```python
from build123d import *

# Parameters (mm, degrees)
SKETCH_1_R          = 8.9
SKETCH_1_R_2        = 1.5
EXTRUDE_1_DEPTH     = 3.5
SKETCH_2_R          = 7.6
CUT_EXTRUDE_1_DEPTH = 0.5
SKETCH_3_R          = 2
EXTRUDE_2_DEPTH     = 13
SKETCH_8_R          = 4
EXTRUDE_4_DEPTH     = 10
CUT_EXTRUDE_START   = -11.5
SKETCH_13_R         = 4
CUT_EXTRUDE_3_DEPTH = 11.5
SKETCH_16_R         = 8.9
SKETCH_16_R_2       = 2
CUT_EXTRUDE_5_DEPTH = 1
SKETCH_17_R         = 2
EXTRUDE_5_DEPTH     = 2


with BuildPart() as part:
    # 草图1 → 凸台-拉伸1 (new body)
    with BuildSketch(Plane.XY):
        Circle(SKETCH_1_R)
        with Locations((0, 5.075)):
            Circle(SKETCH_1_R_2, mode=Mode.SUBTRACT)
        with Locations((4.395078924, -2.5375)):
            Circle(SKETCH_1_R_2, mode=Mode.SUBTRACT)
        with Locations((-4.395078924, -2.5375)):
            Circle(SKETCH_1_R_2, mode=Mode.SUBTRACT)
    extrude(amount=EXTRUDE_1_DEPTH)

    # 草图2 → 切除-拉伸1 (cut)
    with BuildSketch(Plane.XY.offset(3.5)):
        Circle(SKETCH_2_R)
    extrude(amount=-CUT_EXTRUDE_1_DEPTH, mode=Mode.SUBTRACT)

    # 草图3 → 凸台-拉伸2 (add)
    with BuildSketch(Plane(origin=(0, 0, 0), x_dir=(-1, 0, 0), z_dir=(0, 0, -1))):
        with Locations(Location((0, 0, 0), (0, 0, 180))):
            Circle(SKETCH_3_R)
    extrude(amount=EXTRUDE_2_DEPTH)

    # 草图8 → 凸台-拉伸4 (add)
    with BuildSketch(Plane(origin=(0, 0, -8.5), x_dir=(-1, 0, 0), z_dir=(0, 0, -1))):
        Circle(SKETCH_8_R)
    extrude(amount=EXTRUDE_4_DEPTH)

    # 草图13 → 切除-拉伸3 (cut)
    with BuildSketch(Plane(origin=(0, 0, -18.5), x_dir=(-1, 0, 0), z_dir=(0, 0, -1)).offset(CUT_EXTRUDE_START)):
        Circle(SKETCH_13_R)
    extrude(amount=CUT_EXTRUDE_3_DEPTH, mode=Mode.SUBTRACT)

    # 草图16 → 切除-拉伸5 (cut)
    with BuildSketch(Plane(origin=(0, 0, 0), x_dir=(-1, 0, 0), z_dir=(0, 0, -1))):
        Circle(SKETCH_16_R)
        with Locations(Location((0, 0, 0), (0, 0, 180))):
            Circle(SKETCH_16_R_2, mode=Mode.SUBTRACT)
    extrude(amount=-CUT_EXTRUDE_5_DEPTH, mode=Mode.SUBTRACT)

    # 草图17 → 凸台-拉伸5 (add)
    with BuildSketch(Plane(origin=(0, 0, -7), x_dir=(-1, 0, 0), z_dir=(0, 0, -1))):
        with Locations(Location((0, 0, 0), (0, 0, 180))):
            Circle(SKETCH_17_R)
    extrude(amount=EXTRUDE_5_DEPTH)


solid = part.part
```
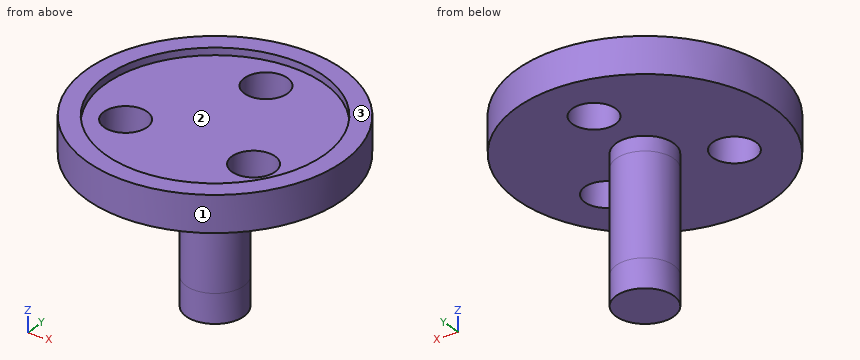
Could you check a few things on this model? Use its own coordinates, in mm. Face numbers are marked on the shaded views. Round coordinates to 2 decimals unless told otherwise and drop trailing zeros. Loops run counter-clockwise (first coordinate to the right, second up) from the corner with the lowest first, then second, coordinate; pieces in that order, holes last. Notation, with made-up numbers: M 29.5,-5 L 63.5,-5 A14 cw 63.5,16 Z; hole C 45,41 d6. An arc over 180 degrees is marked long. Write item = value, one per line.
1. Will these pins go through, and if not, where does the flat tip stop? P1, Ø5, axis at y = -4, z = -6.5, coming from the -X side; P2, Ø6, axis at x = 1.5, z = -3.5, coming from the -Y side; P3, Ø5, axis at x = 4.4, y = -2.54, coming from the -Z side; P4, Ø10, axis at x = -4, y = 0.5, coming from the +Z side.
Results below:
P1 = -1.32
P2 = -2
P3 = 1
P4 = 3.5
2. I want a section at B-B, the plane y = 6. Write out the boundary of the cut face in (x, z), and give its area (3 significant figures).
Results below:
outline = M -6.57,1 L -1.18,1 L -1.18,3 L -4.66,3 L -4.66,3.5 L -6.57,3.5 Z; M 1.18,1 L 6.57,1 L 6.57,3.5 L 4.66,3.5 L 4.66,3 L 1.18,3 Z
area = 23.5 mm²
3. I want a section at D-D, the plane y = 0. Write out the boundary of the cut face in (x, z), and give its area (3 significant figures).
Results below:
outline = M -8.9,1 L -2,1 L -2,-9 L 2,-9 L 2,1 L 8.9,1 L 8.9,3.5 L 7.6,3.5 L 7.6,3 L -7.6,3 L -7.6,3.5 L -8.9,3.5 Z
area = 76.9 mm²
4. Thinking about a two-plate mould opening in X: for the marked faces 1, 2 and 3, which applies, +X half, -X half, draft (parallel to the pull), parting line (faces both ways), or undercut?
Results below:
face_1 = parting line
face_2 = undercut
face_3 = draft
5. I want a section at C-C, the plane y = -3.75. Write out the boundary of the cut face in (x, z), and give its area (3 significant figures).
Results below:
outline = M -8.07,1 L -5.28,1 L -5.28,3 L -6.61,3 L -6.61,3.5 L -8.07,3.5 Z; M -3.51,1 L 3.51,1 L 3.51,3 L -3.51,3 Z; M 5.28,1 L 8.07,1 L 8.07,3.5 L 6.61,3.5 L 6.61,3 L 5.28,3 Z
area = 26.7 mm²
6. I want a section at A-A, the plane x = 0. Write out the boundary of the cut face in (y, z) (3 decimals), and give its area (3 significant figures).
Results below:
outline = M -8.9,1 L -2,1 L -2,-9 L 2,-9 L 2,1 L 3.575,1 L 3.575,3 L -7.6,3 L -7.6,3.5 L -8.9,3.5 Z; M 6.575,1 L 8.9,1 L 8.9,3.5 L 7.6,3.5 L 7.6,3 L 6.575,3 Z
area = 70.9 mm²
7. I need wall thicknesses on probe 1 along Y at (x, z) = (0, 2.2) (3 decimals); probe 2 along Z at (x, y) = (0, -4); probe 3 along Y at (x, z) = (0, 3.35). Which ranges of each line are inside material? Lowest first, please.
Results below:
probe_1 = -8.9 to 3.575, 6.575 to 8.9
probe_2 = 1 to 3
probe_3 = -8.9 to -7.6, 7.6 to 8.9
